The drawing under review shows one solid part. Ordinate dimensions are in mm from its lowest x, y, z. A direction names the side the tool comes from. Round coordinates to 2 decimals unless told otherwise and drop trailing zeros. Loops run counter-clockwise (first coordinate to the right, second up) from the corner with the lowest first, then second, coordinate; pieces in that order, holes last. Notation, with made-up numbers: (42.5, -7.5) - (82.5, -7.5) arc R24 cw to (82.5, 27.5) - close; hole circle Ø1 at (45, 59). An arc over 180 degrees is marked (long way). Answer as CSV lines item,"result".
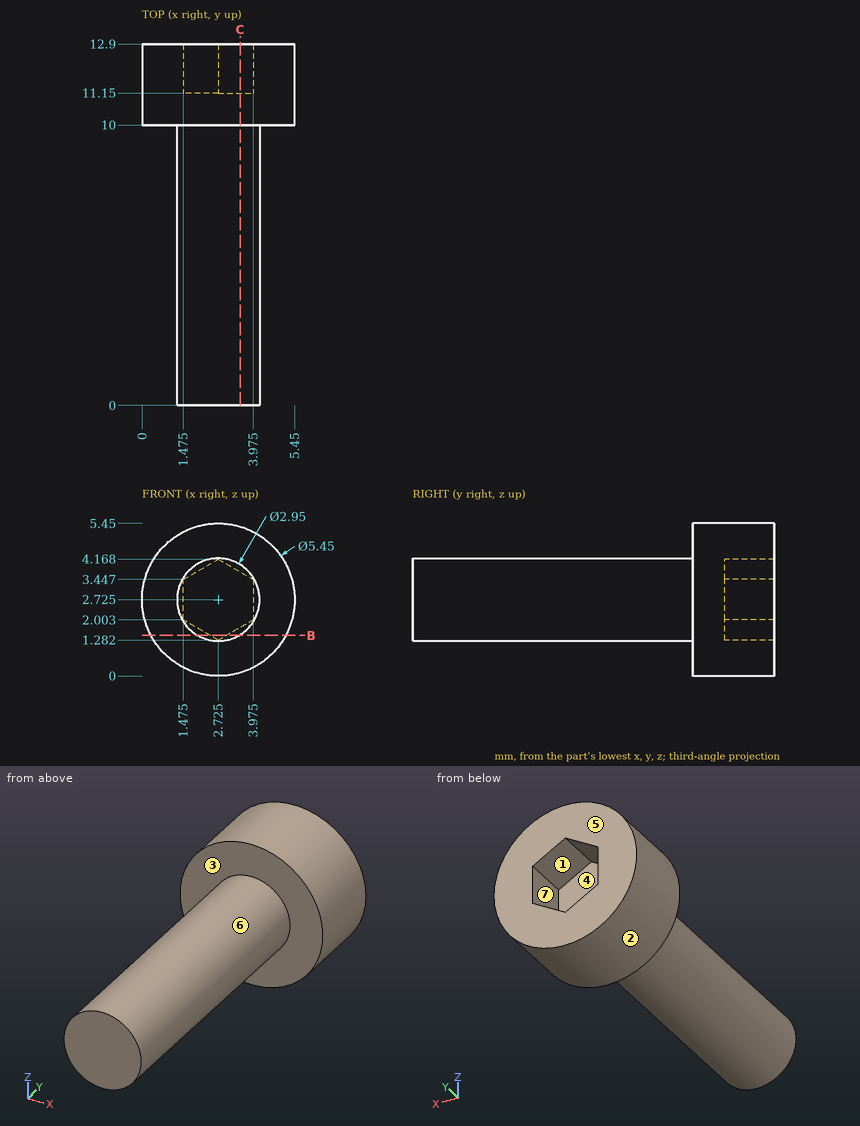
1. Take a section at B-B (z = 1.45). State the section outline as (x, y) points, plus the area to 3 significant figures.
Numbers:
outline,"(0.32, 10) - (1.98, 10) - (1.98, 0) - (3.47, 0) - (3.47, 10) - (5.13, 10) - (5.13, 12.9) - (3.02, 12.9) - (3.02, 11.15) - (2.43, 11.15) - (2.43, 12.9) - (0.32, 12.9) - close"
area,"27.8 mm²"
2. Draft analysis for pull direction X (two halves, no side actions). For the marked faces 1, 2, 3 and 4, state which applies: +X half, -X half, draft (parallel to the pull), parting line (faces both ways), or undercut.
Numbers:
face 1,"undercut"
face 2,"parting line"
face 3,"draft"
face 4,"undercut"
3. Clearance check with flat-ended pins moving along their axes: pin 1 (1 mm diameter, centred on x = 4, y = 3, fed in from +Z); pin 2 (1 mm diameter, centred on y = 11.5, z = 4.5, fed in from -X). State where each tip first meets the part, or that it passes through.
Numbers:
pin 1,"stops at z = 3.98"
pin 2,"stops at x = 0.32"
4. Tool access review of the marked faces 5, 6 and 7: name each direction out of +Z, -Z, +X, -X, +Y, -Y from which nothing blocks a thin tool from reaching the whole face with its end or side.
Numbers:
face 5,"+Z, -Z, +X, -X, +Y"
face 6,"-Y"
face 7,"+Y"
5. Wall thickness on probe 1 along Y at (x, z) = (2, 2.2); probe 2 along Y at (x, z) = (4.45, 1.15); probe 3 along Z at (x, y) = (2.8, 8.5): over which ranges is each line inside the solid? List them lowest first.
Numbers:
probe 1,"y = 0 to 11.15"
probe 2,"y = 10 to 12.9"
probe 3,"z = 1.25 to 4.2"
6. Take a section at C-C (x = 3.5). State the section outline as (y, z) points.
Numbers:
outline,"(0, 1.47) - (10, 1.47) - (10, 0.11) - (12.9, 0.11) - (12.9, 1.73) - (11.15, 1.73) - (11.15, 3.72) - (12.9, 3.72) - (12.9, 5.34) - (10, 5.34) - (10, 3.98) - (0, 3.98) - close"
